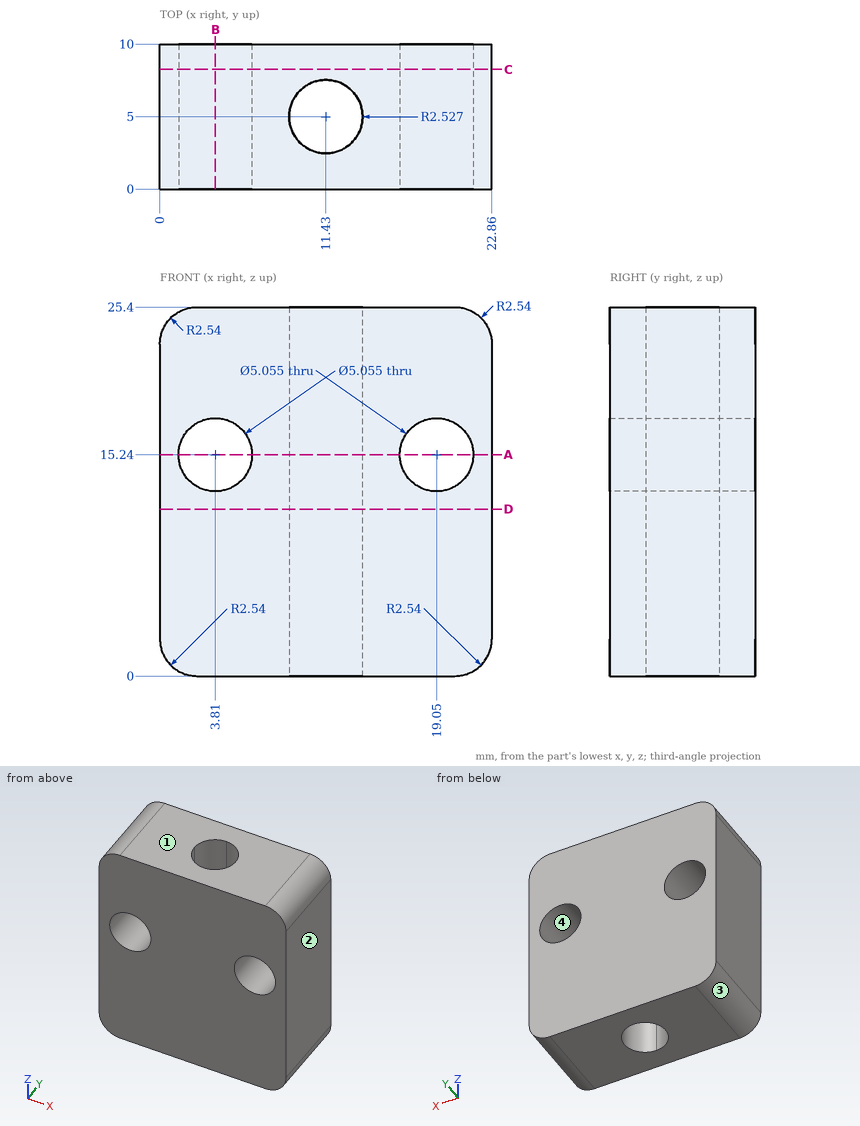
The drawing under review shows one solid part. Ordinate dimensions are in mm from its lowest x, y, z. Coordinates: 2 decimals unless noted, no trailing zeros. Write each loop counter-clockwise with the first axis right and the second up, starting at its lowest first coordinate (ties: lowest second). Pieces come first, ordered by that corner, then holes.
1) Add section B-B (x = 3.81). Write out the cut boundary in (y, z).
2) Add section C-C (y = 8.25). State how many separate pieces and enclosed holes the cut face has, plus the area to 3 significant figures.
3) To check wall thickness, follow L1, parallel to Z at x = 4, y = 8.75; L2, parallel to X at y = 3.75, z = 14.75 (1 decimal); L3, parallel to X at y = 8.25, z = 17 (1 decimal). State the ranges of each line that lie inside material, in increasing order.
4) Add section D-D (z = 11.5). Write out the cut boundary in (x, y) (1 decimal).
5) Add section A-A (z = 15.24). Write out the cut boundary in (x, y) (1 decimal).
6) Insertion check: pin 1 (8 mm diameter, centred on x = 3.81, z = 15.24, fed in from -Y). The pin has a flat end and moves straight along its axis. Give the tip position at first contact, or say it passes through.
7) Mouldability with a two-part tool opening along X and no side actions: class the marked faces 1, 2, 3 and 4 as +X half, -X half, draft (parallel to the pull), parting line (faces both ways), or undercut.
Check result:
1. outline: (0, 0) - (10, 0) - (10, 12.71) - (0, 12.71) - close; (0, 17.77) - (10, 17.77) - (10, 25.4) - (0, 25.4) - close
2. separate pieces: 1
2. enclosed holes: 2
2. area: 535 mm2
3. L1: z = 0 to 12.72, 17.76 to 25.4
3. L2: x = 0 to 1.3, 6.3 to 9.2, 13.6 to 16.6, 21.5 to 22.9
3. L3: x = 0 to 2, 5.6 to 17.2, 20.9 to 22.9
4. outline: (0, 0) - (22.9, 0) - (22.9, 10) - (0, 10) - close; hole circle Ø5.1 at (11.4, 5)
5. outline: (0, 0) - (1.3, 0) - (1.3, 10) - (0, 10) - close; (6.3, 0) - (16.5, 0) - (16.5, 10) - (6.3, 10) - close; (21.6, 0) - (22.9, 0) - (22.9, 10) - (21.6, 10) - close; hole circle Ø5.1 at (11.4, 5)
6. pin 1: stops at y = 0
7. face 1: draft
7. face 2: +X half
7. face 3: -X half
7. face 4: undercut
